Input: part model. Units: mm. Frame: model coordinates. A direction names the side the tool comes from. Give positions to 0.01 mm unless a question says otherwise; leave off trailing zeros. Loops run counter-clockwise (first coordinate to the right, second up) from the corner with the lowest first, then second, coordinate; pieces in that order, holes last.
from build123d import *

# Parameters (mm, degrees)
SKETCH1_R           = 7
BOSS_EXTRUDE1_DEPTH = 19
SKETCH2_R           = 11
BOSS_EXTRUDE2_DEPTH = 223.5
SKETCH3_R           = 7
BOSS_EXTRUDE3_DEPTH = 19
BOSS_EXTRUDE4_START = -3
BOSS_EXTRUDE4_DEPTH = 5.2


with BuildPart() as part:
    # Sketch1 → Boss-Extrude1 (new body)
    with BuildSketch(Plane(origin=(0, 0, 0), x_dir=(1, 0, 0), z_dir=(0, 1, 0))):
        with Locations(Location((0, 0, 0), (0, 0, 270))):
            Circle(SKETCH1_R)
    extrude(amount=BOSS_EXTRUDE1_DEPTH)

    # Sketch2 → Boss-Extrude2 (add)
    with BuildSketch(Plane(origin=(0, 19, 0), x_dir=(1, 0, 0), z_dir=(0, 1, 0))):
        with Locations(Location((0, 0, 0), (0, 0, 270))):
            Circle(SKETCH2_R)
    extrude(amount=BOSS_EXTRUDE2_DEPTH)

    # Sketch3 → Boss-Extrude3 (add)
    with BuildSketch(Plane(origin=(0, 242.5, 0), x_dir=(1, 0, 0), z_dir=(0, 1, 0))):
        with Locations(Location((0, 0, 0), (0, 0, 270))):
            Circle(SKETCH3_R)
    extrude(amount=BOSS_EXTRUDE3_DEPTH)

    # Sketch4 → Boss-Extrude4 (add)
    with BuildSketch(Plane(origin=(7, 0, 0), x_dir=(0, 0, -1), z_dir=(1, 0, 0)).offset(BOSS_EXTRUDE4_START)):
        with BuildLine():
            Line((-2.5, 4.5), (-2.5, 14.5))
            ThreePointArc((-2.5, 14.5), (0, 17), (2.5, 14.5))
            Line((2.5, 14.5), (2.5, 4.5))
            ThreePointArc((2.5, 4.5), (0, 2), (-2.5, 4.5))
        make_face()
    boss_extrude4 = extrude(amount=BOSS_EXTRUDE4_DEPTH)

    # Mirror1: Boss-Extrude4 across plane
    add(boss_extrude4.mirror(Plane.ZX.offset(130.75)))


solid = part.part
(1) Cut plane C-C (y = 87). Return the cut outline in (x, z).
Values follow:
outline: circle Ø22 at (0, 0)
(2) Cut plane B-B (z = 0). Return the cut outline in (x, y).
Values follow:
outline: (-11, 19) - (-7, 19) - (-7, 0) - (7, 0) - (7, 2) - (9.2, 2) - (9.2, 17) - (7, 17) - (7, 19) - (11, 19) - (11, 242.5) - (7, 242.5) - (7, 244.5) - (9.2, 244.5) - (9.2, 259.5) - (7, 259.5) - (7, 261.5) - (-7, 261.5) - (-7, 242.5) - (-11, 242.5) - close
(3) Ray query, probe 1 along Y at (x, z) = (-7.5, 1.5); probe 2 along Z at (x, y) = (-1, 20); probe 3 along Z at (x, y) = (0.5, 17). Return the intervals inside material, ascending.
Values follow:
probe 1: y = 19 to 242.5
probe 2: z = -10.95 to 10.95
probe 3: z = -6.98 to 6.98
(4) Reachability of faces 1 (the flat face through (0, 261.5, 0)), 2 (the flat face through (9.2, 252, 0)), 3 (the flat face through (9.2, 10, 0)) from +Z, -Z, +X, -X, +Y, -Y: full face, straight path, thin tool, end or side. Return the list, or none.
Values follow:
face 1: +Z, -Z, +X, -X, +Y
face 2: +Z, -Z, +X, +Y
face 3: +Z, -Z, +X, -Y
(5) Pin query (flat end, axial travel): pin 1 Ø4 at (y, z) = (251.5, 1) entering from +X; pin 2 Ø2 at (x, y) = (8, 250) entering from -Z; pin 3 Ø6 at (x, y) = (-7.5, 210) entering from +Z. Return the tip coordinate at first contact, or that it passes through.
Values follow:
pin 1: stops at x = 9.2
pin 2: stops at z = -2.5
pin 3: stops at z = 10.04
(6) Cut plane A-A (x = 0). Return the cut outline in (y, z).
Values follow:
outline: (0, -7) - (19, -7) - (19, -11) - (242.5, -11) - (242.5, -7) - (261.5, -7) - (261.5, 7) - (242.5, 7) - (242.5, 11) - (19, 11) - (19, 7) - (0, 7) - close
